```python
from build123d import *

# Parameters (mm, degrees)
SKETCH1_R           = 22.7
SKETCH1_R_2         = 10.5
BOSS_EXTRUDE1_DEPTH = 6
SKETCH2_OUTSIDE_W   = 60.464
SKETCH2_OUTSIDE_H   = 60.464
SKETCH2_OUTSIDE_R   = 15.8
CUT_EXTRUDE1_DEPTH  = 2.5
FILLET1_R           = 6
CUT_EXTRUDE2_DEPTH  = 34.478799262
CIRPATTERN1_COUNT   = 16


with BuildPart() as part:
    # Sketch1 → Boss-Extrude1 (new, symmetric)
    with BuildSketch(Plane(origin=(0, 0, 0), x_dir=(1, 0, 0), z_dir=(0, 1, 0))):
        with Locations(Location((0, 0, 0), (0, 0, 270))):
            Circle(SKETCH1_R)
        with Locations(Location((0, 0, 0), (0, 0, 270))):
            Circle(SKETCH1_R_2, mode=Mode.SUBTRACT)
    extrude(amount=BOSS_EXTRUDE1_DEPTH, both=True)

    # Sketch2 outside → Cut-Extrude1 (cut)
    with BuildSketch(Plane(origin=(0, 6, 0), x_dir=(1, 0, 0), z_dir=(0, 1, 0))):
        Rectangle(SKETCH2_OUTSIDE_W, SKETCH2_OUTSIDE_H)
        with Locations(Location((0, 0, 0), (0, 0, 270))):
            Circle(SKETCH2_OUTSIDE_R, mode=Mode.SUBTRACT)
    cut_extrude1 = extrude(amount=-CUT_EXTRUDE1_DEPTH, mode=Mode.SUBTRACT)

    # Mirror1: Cut-Extrude1 across plane
    add(cut_extrude1.mirror(Plane.ZX), mode=Mode.SUBTRACT)

    # Fillet1
    # the kernel refuses this fillet: 6 mm, written as the material it adds along each edge
    with BuildSketch(Plane(origin=(0, -3.5, 0), x_dir=(0, 0, 1), z_dir=(-1, 0, 0))) as fillet1_piece_1:
        with BuildLine():
            CenterArc((20.673397172, -6), FILLET1_R, 90, 54.314665287)
            Line((15.8, -2.5), (15.702532057, -2.43))
            ThreePointArc((15.702532057, -2.43), (15.68, -1.25), (15.68, 0))
            Line((15.68, 0), (15.8, 0.12))
            Line((15.8, 0.12), (20.673397172, 0.12))
            Line((20.673397172, 0.12), (20.673397172, 0))
        make_face()
    revolve(axis=Axis((0, -3.5, 0), (0, 1, 0)))

    # Sketch3 → Cut-Extrude2 (cut, through all)
    with BuildSketch(Plane.XZ.offset(3.5)):
        with BuildLine():
            ThreePointArc((-2.779777309, 21.823745819), (0, 20.7), (2.779777309, 21.823745819))
            ThreePointArc((2.779777309, 21.823745819), (3.498507516, 22.243201944), (4.329718774, 22.283256839))
            ThreePointArc((4.329718774, 22.283256839), (0, 22.7), (-4.329718774, 22.283256839))
            ThreePointArc((-4.329718774, 22.283256839), (-3.498507516, 22.243201944), (-2.779777309, 21.823745819))
        make_face()
    cut_extrude2 = extrude(amount=-CUT_EXTRUDE2_DEPTH, mode=Mode.SUBTRACT)

    # CirPattern1: Cut-Extrude2 ×16 about axis
    cirpattern1_axis = Axis((0, 0, 0), (0, 1, 0))
    for i in range(1, CIRPATTERN1_COUNT):
        add(cut_extrude2.rotate(cirpattern1_axis, i * 360 / CIRPATTERN1_COUNT), mode=Mode.SUBTRACT)


solid = part.part
```
Verification items for the finished model (mm, model axes). Round coordinates to 2 decimals unless told otherwise and drop trailing zeros. Write each loop counter-clockwise with the first axis right and the second up, starting at its lowest first coordinate (ties: lowest second). Pieces come first, ordered by that corner, then holes. Notation, with made-up numbers: (27, 27.5) - (77, 27.5) arc R13 ccw to (77, 51.5) - close; hole circle Ø1 at (41, 51). An arc over 180 degrees is marked (long way). Answer as a JSON object with one key per item and string values. Group by question number.
Q1. Mould release check, pull along X, two halves, no side actions. Record for faces 1 (the cylindrical face through (19.11, -0.05, 7.96)), 2 (the flat face through (7, 3.5, -15)), 3 (the cylindrical face through (-13.25, -0.05, -18.21)), 4 (the cylindrical face through (3.51, -0.049, -22.247)): released by +X, released by -X, zero draft, split by the parting line, or undercut.
Q2. Thickness scan on line 1 (X direction, y = 0.5, z = 0.5); line 2 (X direction, y = -3.25, z = -3.5); line 3 (Z direction, x = -5, y = 4.75). Record the ranges inside material, lowest first.
Q3. Section check C-C, the plane y = -5. Enter the section's corners in (x, z), plus the area to 3 significant figures.
Q4. Go/stop test with flat-tipped pins: pin 1 Ø6 at (y, z) = (1, -7.5) entering from -X; pin 2 Ø6 at (x, y) = (11.5, -4) entering from -Z; pin 3 Ø5 at (x, y) = (-15, 3.5) entering from -Z. Record where each tip stops, or that it passes through.
Found:
{
 "1": {"face 1": "released by +X", "face 2": "zero draft", "face 3": "released by -X", "face 4": "undercut"},
 "2": {"line 1": "x = -20.73 to -10.49, 10.49 to 20.73", "line 2": "x = -22.24 to -9.9, 9.9 to 22.24", "line 3": "z = -14.99 to -9.23, 9.23 to 14.99"},
 "3": {"outline": "circle Ø33.41 at (0, 0); hole circle Ø21 at (0, 0)", "area": "530 mm^2"},
 "4": {"pin 1": "stops at x = -22.25", "pin 2": "stops at z = -19.22", "pin 3": "stops at z = -18.95"}
}
